The listing builds one solid part. Answer for the finished solid, in the listing's coordinates (mm). A direction names the side the tool comes from. Coordinates: 2 decimals unless noted, no trailing zeros. Order: outer loops, then holes, each group sorted by start corner. A loop starts at its lowest first (then second) coordinate and runs counter-clockwise, first axis right, second up.
from build123d import *

# Parameters (mm, degrees)
PAD_DEPTH       = 10
POCKET_DEPTH    = 8
PAD001_DEPTH    = 10
POCKET001_DEPTH = 10.001
SKETCH004_W     = 160
SKETCH004_H     = 60
PAD002_DEPTH    = 10
SKETCH005_W     = 156
SKETCH005_H     = 56
POCKET002_DEPTH = 8
SKETCH006_W     = 18
SKETCH006_H     = 12
POCKET003_DEPTH = 8


with BuildPart() as part:
    # Sketch001 → Pad (new body)
    with BuildSketch(Plane.XY):
        with BuildLine():
            ThreePointArc((0, 57.236352), (-106.486482, 50.845622), (-101.68, -55.72412))
            Line((-101.68, -55.72412), (0, -150.0248))
            Line((0, -150.0248), (101.68, -55.72412))
            ThreePointArc((101.68, -55.72412), (106.486482, 50.845622), (0, 57.236352))
        make_face()
    extrude(amount=PAD_DEPTH)

    # Sketch002 → Pocket (cut)
    with BuildSketch(Plane.XY.offset(10)):
        with BuildLine():
            ThreePointArc((0, 54.552727), (-104.405447, 50.160217), (-100.32, -54.257696))
            Line((-100.32, -54.257696), (0, -147.297076))
            Line((0, -147.297076), (100.32, -54.257696))
            ThreePointArc((100.32, -54.257696), (104.405447, 50.160217), (0, 54.552727))
        make_face()
    extrude(amount=-POCKET_DEPTH, mode=Mode.SUBTRACT)

    # Sketch003 → Pad001 (join)
    with BuildSketch(Plane.XY):
        with BuildLine():
            ThreePointArc((0, 29.393877), (-86.345652, 45.199486), (-89.44, -42.526302))
            Line((-89.44, -42.526302), (0, -125.475287))
            Line((0, -125.475287), (89.44, -42.526302))
            ThreePointArc((89.44, -42.526302), (86.345652, 45.199486), (0, 29.393877))
        make_face()
    extrude(amount=PAD001_DEPTH)

    # Sketch → Pocket001 (cut, through all)
    with BuildSketch(Plane.XY.offset(10)):
        with BuildLine():
            ThreePointArc((0, 25.21904), (-83.671135, 44.74656), (-88.08, -41.059878))
            Line((-88.08, -41.059878), (0, -122.747563))
            Line((0, -122.747563), (88.08, -41.059878))
            ThreePointArc((88.08, -41.059878), (83.671135, 44.74656), (0, 25.21904))
        make_face()
    extrude(amount=-POCKET001_DEPTH, mode=Mode.SUBTRACT)

    # Sketch004 → Pad002 (join)
    with BuildSketch(Plane.XY):
        with Locations((0, -170)):
            Rectangle(SKETCH004_W, SKETCH004_H)
    extrude(amount=PAD002_DEPTH)

    # Sketch005 → Pocket002 (cut)
    with BuildSketch(Plane.XY.offset(10)):
        with Locations((0, -170)):
            Rectangle(SKETCH005_W, SKETCH005_H)
    extrude(amount=-POCKET002_DEPTH, mode=Mode.SUBTRACT)

    # Sketch006 → Pocket003 (cut)
    with BuildSketch(Plane.XY.offset(10)):
        with Locations((0, -140.2931)):
            Rectangle(SKETCH006_W, SKETCH006_H)
    extrude(amount=-POCKET003_DEPTH, mode=Mode.SUBTRACT)


solid = part.part
(1) Find the intervals of material crossed by probe 1 along X at (y, z) = (0, 4.75); probe 2 along X at (y, z) = (-143, 9); probe 3 along X at (y, z) = (-140.5, 3.5), in increasing order.
(2) Find section A-A on y = 0. Determine the outline of the cut face in (x, z), then the cut area to 3 significant figures.
(3) A tool of negligible diameter and unlimited length cuts with its end or side. For faces 1 (the flat face through (-78, -170, 6)), 2 (the flat face through (43.4, -82.5, 5.1)), 3 (the flat face through (-56.881, -97.272, 4.93)), from which of +Z, -Z, +X, -X, +Y, -Y can it reach the whole face along a straight path? Write none if from no direction.
(4) The mould has two halves that part along Y. Classify faces 4 (the flat face through (80, -170, 5)), 5 (the cylindrical face through (87.421, 44.313, 5.944)): pulls with the +Y half, pulls with the -Y half, needs draft (parallel to the pull), parting line crosses it, or undercut.
(5) Find section B-B on z = 5.75. Determine the outline of the cut face in (x, y).
(6) Find section C-C on x = -29. Determine the outline of the cut face in (y, z).
(7) Given pin 1 Ø5 at (y, z) = (-165, 7) entering from +X; pin 2 Ø12 at (x, y) = (-24.5, -133) entering from +Z; pin 3 Ø0.9 at (y, z) = (-140.5, 7) entering from -X; pin 4 Ø3 at (y, z) = (-126.5, 8) entering from -X, each flat-ended and moving along its own axis, determine where each tip first touches the part or whether it passes through.
(8) Find section D-D on x = 3. Determine the outline of the cut face in (y, z), then the cut area to 3 significant figures.
Resolved:
1. probe 1: x = -126 to -124, -108 to -106, 106 to 108, 124 to 126
1. probe 2: x = -80 to -78, 78 to 80
1. probe 3: x = -80 to -9, 9 to 80
2. outline: (-126, 0) - (-106, 0) - (-106, 10) - (-108, 10) - (-108, 2) - (-124, 2) - (-124, 10) - (-126, 10) - close; (106, 0) - (126, 0) - (126, 10) - (124, 10) - (124, 2) - (108, 2) - (108, 10) - (106, 10) - close
2. area: 144 mm2
3. face 1: +Z
3. face 2: +Z, -Z
3. face 3: +Z, -Z, -X
4. face 4: needs draft
4. face 5: undercut
5. outline: (-101.68, -55.72) - (-10.81, -140) - (-80, -140) - (-80, -200) - (80, -200) - (80, -140) - (10.81, -140) - (101.68, -55.72) arc R76 ccw to (0, 57.24) arc R76 ccw to start; (-89.44, -42.53) - (0, -125.48) - (89.44, -42.53) arc R58 ccw (long way) to (0, 29.39) arc R58 ccw (long way) to start; hole (-100.32, -54.26) - (-9, -138.95) - (-9, -142) - (-78, -142) - (-78, -198) - (78, -198) - (78, -142) - (9, -142) - (9, -138.95) - (100.32, -54.26) arc R74 ccw to (0, 54.55) arc R74 ccw to start; hole (-88.08, -41.06) - (0, -122.75) - (88.08, -41.06) arc R56 ccw (long way) to (0, 25.22) arc R56 ccw (long way) to start
6. outline: (-200, 0) - (-140, 0) - (-140, 10) - (-142, 10) - (-142, 2) - (-198, 2) - (-198, 10) - (-200, 10) - close; (-123.13, 0) - (-95.85, 0) - (-95.85, 10) - (-98.58, 10) - (-98.58, 2) - (-120.4, 2) - (-120.4, 10) - (-123.13, 10) - close; (51.91, 0) - (73.04, 0) - (73.04, 10) - (70.96, 10) - (70.96, 2) - (54.06, 2) - (54.06, 10) - (51.91, 10) - close
7. pin 1: stops at x = 80
7. pin 2: stops at z = 10
7. pin 3: stops at x = -80
7. pin 4: stops at x = -26.98
8. outline: (-200, 0) - (-119.97, 0) - (-119.97, 10) - (-122.69, 10) - (-122.69, 2) - (-198, 2) - (-198, 10) - (-200, 10) - close; (30.45, 0) - (59.72, 0) - (59.72, 10) - (57.16, 10) - (57.16, 2) - (33.99, 2) - (33.99, 10) - (30.45, 10) - close
8. area: 305 mm2
